```python
from build123d import *

# Parameters (mm, degrees)
BOSS_EXTRU_1_DEPTH      = 2
ESQUISSE2_W             = 2
ESQUISSE2_H             = 43.4
BOSS_EXTRU_2_DEPTH      = 23
ESQUISSE3_W             = 2
ESQUISSE3_H             = 23
BOSS_EXTRU_3_DEPTH      = 8
ESQUISSE8_W             = 2
ESQUISSE8_H             = 23
BOSS_EXTRU_5_DEPTH      = 8
ESQUISSE9_R             = 2
ENL_V_MAT_EXTRU_3_DEPTH = 2
ESQUISSE10_R            = 1.5
ESQUISSE10_R_2          = 2.25
ENL_V_MAT_EXTRU_4_DEPTH = 2
ENL_V_MAT_EXTRU_5_REACH = 47.66
ESQUISSE11_R            = 2.1
ESQUISSE13_R            = 2.65
BOSS_EXTRU_6_DEPTH      = 43.4
ENL_V_MAT_EXTRU_6_DEPTH = 10
ENL_V_MAT_EXTRU_7_DEPTH = 10
CHANFREIN1_SIZE         = 2
CHANFREIN2_SIZE         = 2


with BuildPart() as part:
    # Esquisse1 → Boss.-Extru.1 (new body)
    with BuildSketch(Plane.XY):
        Polygon((8.75, 17), (8.75, 19), (13.75, 19), (13.75, 27), (-10.25, 27), (-10.25, 19), (-20.25, 19), (-20.25, -24.4), (-10.25, -24.4), (-10.25, -32.4), (13.75, -32.4), (13.75, -24.4), (8.75, -24.4), (8.75, -22.4), (16.25, -22.4), (16.25, 17), align=None)
    extrude(amount=BOSS_EXTRU_1_DEPTH)

    # Esquisse2 → Boss.-Extru.2 (add)
    with BuildSketch(Plane(origin=(0, 0, 0), x_dir=(-1, 0, 0), z_dir=(0, 0, -1))):
        with Locations((19.25, -2.7)):
            Rectangle(ESQUISSE2_W, ESQUISSE2_H)
    extrude(amount=BOSS_EXTRU_2_DEPTH)

    # Esquisse3 → Boss.-Extru.3 (add)
    with BuildSketch(Plane(origin=(0, 27, 0), x_dir=(1, 0, 0), z_dir=(0, 1, 0))):
        with Locations((12.75, 11.5)):
            Rectangle(ESQUISSE3_W, ESQUISSE3_H)
    extrude(amount=-BOSS_EXTRU_3_DEPTH)

    # Esquisse8 → Boss.-Extru.5 (add)
    with BuildSketch(Plane.XZ.offset(32.4)):
        with Locations((12.75, -11.5)):
            Rectangle(ESQUISSE8_W, ESQUISSE8_H)
    extrude(amount=-BOSS_EXTRU_5_DEPTH)

    # Esquisse9 → Enlèv. mat.-Extru.3 (cut)
    with BuildSketch(Plane(origin=(13.75, 0, 0), x_dir=(0, 0, -1), z_dir=(1, 0, 0))):
        with Locations((6, 22.5)):
            Circle(ESQUISSE9_R)
        with Locations((16, 22.5)):
            Circle(ESQUISSE9_R)
        with Locations(Location((16, -27.9, 0), (0, 0, 180))):
            Circle(ESQUISSE9_R)
        with Locations(Location((6, -27.9, 0), (0, 0, 180))):
            Circle(ESQUISSE9_R)
    extrude(amount=-ENL_V_MAT_EXTRU_3_DEPTH, mode=Mode.SUBTRACT)

    # Esquisse10 → Enlèv. mat.-Extru.4 (cut)
    with BuildSketch(Plane.ZY.offset(20.25)):
        with Locations((-11, 14.1)):
            Circle(ESQUISSE10_R)
        with Locations((-11, 7.1)):
            Circle(ESQUISSE10_R_2)
        with Locations((-4, 7.1)):
            Circle(ESQUISSE10_R)
        with Locations((-11, 0.1)):
            Circle(ESQUISSE10_R)
        with Locations((-18, 7.1)):
            Circle(ESQUISSE10_R)
        with Locations(Location((-11, -5.5, 0), (0, 0, 180))):
            Circle(ESQUISSE10_R)
        with Locations(Location((-11, -12.5, 0), (0, 0, 180))):
            Circle(ESQUISSE10_R_2)
        with Locations(Location((-4, -12.5, 0), (0, 0, 180))):
            Circle(ESQUISSE10_R)
        with Locations(Location((-18, -12.5, 0), (0, 0, 180))):
            Circle(ESQUISSE10_R)
        with Locations(Location((-11, -19.5, 0), (0, 0, 180))):
            Circle(ESQUISSE10_R)
    extrude(amount=-ENL_V_MAT_EXTRU_4_DEPTH, mode=Mode.SUBTRACT)

    # Esquisse11 → Enlèv. mat.-Extru.5 (cut, up to next)
    with BuildSketch(Plane.XY.offset(2), mode=Mode.PRIVATE) as enl_v_mat_extru_5_sk1:
        with Locations((-6.25, 23)):
            Circle(ESQUISSE11_R)
    enl_v_mat_extru_5_tool1 = extrude(enl_v_mat_extru_5_sk1.sketch, amount=-ENL_V_MAT_EXTRU_5_REACH, mode=Mode.PRIVATE) & part.part
    # Esquisse11 → Enlèv. mat.-Extru.5 (cut, up to next)
    with BuildSketch(Plane.XY.offset(2), mode=Mode.PRIVATE) as enl_v_mat_extru_5_sk2:
        with Locations((4.75, 23)):
            Circle(ESQUISSE11_R)
    enl_v_mat_extru_5_tool2 = extrude(enl_v_mat_extru_5_sk2.sketch, amount=-ENL_V_MAT_EXTRU_5_REACH, mode=Mode.PRIVATE) & part.part
    # Esquisse11 → Enlèv. mat.-Extru.5 (cut, up to next)
    with BuildSketch(Plane.XY.offset(2), mode=Mode.PRIVATE) as enl_v_mat_extru_5_sk3:
        with Locations((4.75, -28.4)):
            Circle(ESQUISSE11_R)
    enl_v_mat_extru_5_tool3 = extrude(enl_v_mat_extru_5_sk3.sketch, amount=-ENL_V_MAT_EXTRU_5_REACH, mode=Mode.PRIVATE) & part.part
    # Esquisse11 → Enlèv. mat.-Extru.5 (cut, up to next)
    with BuildSketch(Plane.XY.offset(2), mode=Mode.PRIVATE) as enl_v_mat_extru_5_sk4:
        with Locations((-6.25, -28.4)):
            Circle(ESQUISSE11_R)
    enl_v_mat_extru_5_tool4 = extrude(enl_v_mat_extru_5_sk4.sketch, amount=-ENL_V_MAT_EXTRU_5_REACH, mode=Mode.PRIVATE) & part.part
    add(enl_v_mat_extru_5_tool1.solids().sort_by_distance((-6.25, 23, 2))[0], mode=Mode.SUBTRACT)
    add(enl_v_mat_extru_5_tool2.solids().sort_by_distance((4.75, 23, 2))[0], mode=Mode.SUBTRACT)
    add(enl_v_mat_extru_5_tool3.solids().sort_by_distance((4.75, -28.4, 2))[0], mode=Mode.SUBTRACT)
    add(enl_v_mat_extru_5_tool4.solids().sort_by_distance((-6.25, -28.4, 2))[0], mode=Mode.SUBTRACT)

    # Esquisse13 → Boss.-Extru.6 (add)
    # profile 1 of 2: a face of its own
    with BuildSketch(Plane.XZ.offset(24.4)):
        with BuildLine():
            Line((-10.25, 0), (-20.25, 0))
            Line((-20.25, 0), (-20.25, 7))
            ThreePointArc((-20.25, 7), (-15.25, 12), (-10.25, 7))
            Line((-10.25, 7), (-10.25, 0))
        make_face()
        with Locations(Location((-15.25, 7, 0), (0, 0, 270))):
            Circle(ESQUISSE13_R, mode=Mode.SUBTRACT)
    # profile 2 of 2: a face of its own
    with BuildSketch(Plane.XZ.offset(24.4)):
        with BuildLine():
            Line((8.75, 0), (18.75, 0))
            Line((18.75, 0), (18.75, 7))
            ThreePointArc((18.75, 7), (13.75, 12), (8.75, 7))
            Line((8.75, 7), (8.75, 0))
        make_face()
        with Locations(Location((13.75, 7, 0), (0, 0, 270))):
            Circle(ESQUISSE13_R, mode=Mode.SUBTRACT)
    extrude(amount=-BOSS_EXTRU_6_DEPTH)

    # Esquisse14 → Enlèv. mat.-Extru.6 (cut)
    with BuildSketch(Plane(origin=(0, 19, 0), x_dir=(1, 0, 0), z_dir=(0, 1, 0))):
        Polygon((-10.25, -2), (-20.25, -2), (-20.25, 7.294749089), (-22.778908198, 7.294749089), (-22.778908198, -2), (-24.693194377, -2), (-24.693194377, -14.280851393), (-10.25, -14.280851393), align=None)
        Polygon((8.75, -2), (13.75, -2), (13.75, 5.181058099), (21.169912006, 5.181058099), (21.169912006, -2), (27.112175355, -2), (27.112175355, -13.044541568), (8.75, -13.044541568), align=None)
    extrude(amount=-ENL_V_MAT_EXTRU_6_DEPTH, mode=Mode.SUBTRACT)

    # Esquisse15 → Enlèv. mat.-Extru.7 (cut)
    with BuildSketch(Plane.XZ.offset(24.4)):
        Polygon((-7.765139989, 2), (-20.25, 2), (-20.25, -7.221906492), (-27.573956422, -7.221906492), (-27.573956422, 2), (-33.179445784, 2), (-33.179445784, 15.314448699), (-7.765139989, 15.314448699), align=None)
        Polygon((6.630968462, 2), (13.75, 2), (13.75, -6.0207302), (22.303459128, -6.0207302), (22.303459128, 2), (24.534215098, 2), (24.534215098, 15.314448699), (6.630968462, 15.314448699), align=None)
    extrude(amount=-ENL_V_MAT_EXTRU_7_DEPTH, mode=Mode.SUBTRACT)

    # Chanfrein1
    # the kernel refuses this chamfer: 2 mm, written as the material it takes off along each edge
    with BuildSketch(Plane(origin=(18.893365976, 27, 2), x_dir=(0, -0.9996219169112968, 0.027495876610586296), z_dir=(-1, 0, 0))) as chanfrein1_piece_1:
        Polygon((CHANFREIN1_SIZE * 0.999621916911, -CHANFREIN1_SIZE * 0.0274958766106), (-CHANFREIN1_SIZE * 0.0274958766106, -CHANFREIN1_SIZE * 0.999621916911), (0, 0), align=None)
    extrude(amount=34.286731952, mode=Mode.SUBTRACT)

    # Chanfrein2
    # the kernel refuses this chamfer: 2 mm, written as the material it takes off along each edge
    with BuildSketch(Plane(origin=(-15.393365976, -32.4, 2), x_dir=(0, -0.02749587661058563, -0.9996219169112968), z_dir=(1, 0, 0))) as chanfrein2_piece_1:
        Polygon((CHANFREIN2_SIZE * 0.999621916911, CHANFREIN2_SIZE * 0.0274958766106), (-CHANFREIN2_SIZE * 0.0274958766106, CHANFREIN2_SIZE * 0.999621916911), (0, 0), align=None)
    extrude(amount=34.286731952, mode=Mode.SUBTRACT)


solid = part.part
```
The model under review builds one solid part; all positions refer to its coordinate system, in mm. A direction names the side the tool comes from. Round coordinates to 2 decimals unless told otherwise and drop trailing zeros. Write each loop counter-clockwise with the first axis right and the second up, starting at its lowest first coordinate (ties: lowest second). Pieces come first, ordered by that corner, then holes.
(1) We need section D-D on x = 10. Give the boundary of the cut face in (y, z).
(2) We need section B-B on x = 4.75. Give the boundary of the cut face in (y, z), and give its area (3 significant figures).
(3) We need section A-A on y = -5.5. Give the boundary of the cut face in (x, z).
(4) Mouldability with a two-part tool opening along Y and no side actions: class faces 1 (the cylindrical face through (-6.523, -26.318, 1.014)), 2 (the flat face through (1.6, -31.4, 1)), 3 (the cylindrical face through (-15.133, -2.864, 9.647)), 4 (the cylindrical face through (12.764, -25.948, -16.434)) as +Y half, -Y half, draft (parallel to the pull), parting line (faces both ways), or undercut.
(5) We need section C-C on y = 7.1. Give the boundary of the cut face in (x, z).
(6) Wall thickness on L1, parallel to Y at x = 12, z = -19.5; L2, parallel to Y at x = 12.9, z = -16; L3, parallel to Z at x = -19.8, y = -12.5: over which ranges is each line inside the solid? List them lowest first.
(7) Machinability: for faces 5 (the flat face through (-10.25, -3, 5)), 6 (the flat face through (-18.25, -3, -11)), 7 (the flat face through (-10.25, 22, 1)), which of the approach directions +Z, -Z, +X, -X, +Y, -Y give a long, thin tool a straight path to every point of the face, cutting with its end or side? Answer none if there is none.
(8) Insertion check: pin 1 (5 mm diameter, centred on x = 16, z = 3, fed in from -Y); pin 2 (8 mm diameter, centred on x = 4.5, y = -4.5, fed in from +Z); pin 3 (6.5 mm diameter, centred on y = 22.5, z = -6, fed in from -X); pin 4 (5 mm diameter, centred on x = -14.5, z = -7.5, fed in from +Y). Each pin has a flat end and moves straight along its axis. Give the tip position at first contact, or say it passes through.
Findings below:
1. outline: (-32.4, 0) - (27, 0) - (25, 2) - (9, 2) - (9, 10.31) - (-14.4, 10.31) - (-14.4, 2) - (-30.4, 2) - close
2. outline: (-32.4, 0) - (-30.5, 0) - (-30.5, 1.9) - close; (-26.3, 0) - (20.9, 0) - (20.9, 2) - (-26.3, 2) - close; (25.1, 0) - (27, 0) - (25.1, 1.9) - close
2. area: 98.0 mm2
3. outline: (-20.25, -23) - (-18.25, -23) - (-18.25, -12.5) - (-20.25, -12.5) - close; (-20.25, -9.5) - (-18.25, -9.5) - (-18.25, 0) - (18.75, 0) - (18.75, 7) arc R5 ccw to (8.75, 7) - (8.75, 2) - (-10.25, 2) - (-10.25, 7) arc R5 ccw to (-20.25, 7) - close; hole circle Ø5.3 at (-15.25, 7); hole circle Ø5.3 at (13.75, 7)
4. face 1: undercut
4. face 2: -Y half
4. face 3: draft
4. face 4: undercut
5. outline: (-20.25, -23) - (-18.25, -23) - (-18.25, -19.5) - (-20.25, -19.5) - close; (-20.25, -16.5) - (-18.25, -16.5) - (-18.25, -13.25) - (-20.25, -13.25) - close; (-20.25, -8.75) - (-18.25, -8.75) - (-18.25, -5.5) - (-20.25, -5.5) - close; (-20.25, -2.5) - (-18.25, -2.5) - (-18.25, 0) - (18.75, 0) - (18.75, 7) arc R5 ccw to (8.75, 7) - (8.75, 2) - (-10.25, 2) - (-10.25, 7) arc R5 ccw to (-20.25, 7) - close; hole circle Ø5.3 at (-15.25, 7); hole circle Ø5.3 at (13.75, 7)
6. L1: y = -32.4 to -24.4, 19 to 27
6. L2: y = -32.4 to -29.9, -25.9 to -24.4, 19 to 20.5, 24.5 to 27
6. L3: z = -23 to -19.5, -16.5 to -13.25, -8.75 to -5.5, -2.5 to 9.07
7. face 5: +Z, +Y, -Y
7. face 6: -Z, +X, +Y, -Y
7. face 7: +Z, -Z, -X, +Y
8. pin 1: stops at y = -30.49
8. pin 2: stops at z = 2
8. pin 3: stops at x = 11.75
8. pin 4: passes through
